Input: part model. Units: mm. Frame: model coordinates. A direction names the side the tool comes from. Coordinates: 2 decimals unless noted, no trailing zeros. Loops run counter-clockwise (first coordinate to the right, second up) from the corner with the lowest first, then second, coordinate; pieces in that order, holes last. Notation, with made-up numbers: (13.25, 4.5) - (68.25, 4.5) arc R23 ccw to (68.25, 26.5) - close; hole circle Ø2 at (-27, -38). An arc over 180 degrees is marked (long way). Use a Markdown table: item, result. Add a question column.
1. Contact query for flat-ended pins moving along their axis: P1, Ø24, axis at x = -31, y = 1.5, coming from the -Z side; P2, Ø2.5, axis at x = -37, y = -3.5, coming from the +Z side; P3, Ø15, axis at y = -4, z = 15.5, coming from the +X side. Output: stop coordinate, or through.
2. Access query for faces 4 (the face through (-39.65, 0.07, 1.01)), 5 (the face through (-22, 0, 2)), 6 (the face through (-30.182, -22.395, 1.014)), 7 (the face through (-35.35, -3.43, 52.99)). Directions: +Z, -Z, +X, -X, +Y, -Y. A direction counts if a zero-diameter tool reaches every point of the face in a straight line with its end or side. Return the directions, or none.
3. Section query B-B on y = -9. Return the cut outline in (x, z), then the cut area to 3 significant figures.
4. Draft query along Z for faces 1 (the face through (-4.69, -8, 1.01)), 2 (the face through (-22, 0, 54)), 3 (the face through (-22, 0, 52)). Return one class per face: released by +Z, released by -Z, zero draft, split by the parting line, or undercut.
5. Section query A-A on x = -2.5. Return the cut outline in (y, z), then the cut area to 3 significant figures.
6. Ray query, L1, parallel to Y at x = -6, z = 1; L2, parallel to Y at x = -37, z = 53; L3, parallel to Z at x = -9, y = 4. Return the intervals inside material, ascending. Write a range as [from, to].
7. Section query D-D on z = 19.5. Return the cut outline in (x, y).
8. Section query C-C on y = 23. Return the cut outline in (x, z).
```python
from build123d import *

# Parameters (mm, degrees)
F1_DEPTH  = 15
F3_D      = 3.3
F5_D      = 3.3
F5_DEPTH  = 13.5
F5_TIP    = 0.9914200214
F7_D      = 3.3
F7_DEPTH  = 13.5
F7_TIP    = 0.9914200214
F9_DEPTH  = 2
F12_D     = 3.3
F12_DEPTH = 13.5
F12_TIP   = 0.9914200214


with BuildPart() as f1:
    # F0 (on Front) → F1 (new body, symmetric)
    with BuildSketch(Plane.XZ):
        Polygon((-45, 0), (0, 0), (0, 2), (-43, 2), (-43, 52), (0, 52), (0, 54), (-45, 54), align=None)
    extrude(amount=F1_DEPTH, both=True)

    # F3 (through all)
    with Locations(Plane(origin=(0, 0, 0), x_dir=(1, 0, 0), z_dir=(0, 0, -1))):
        with Locations((-6, 9), (-6, -9)):
            Hole(F3_D / 2)

    # F5
    with Locations(Plane.XY.offset(54)):
        with Locations((-37, 3.5), (-37, -3.5)):
            Hole(F5_D / 2, depth=F5_DEPTH)
            with Locations((0, 0, -(F5_DEPTH + F5_TIP / 2))):  # 118° drill point
                Cone(0, F5_D / 2, F5_TIP, mode=Mode.SUBTRACT)

    # F7 (one way)
    with BuildSketch(Plane.XY.offset(2)):
        with Locations((-37.9999987781, 0)):
            Circle(F7_D / 2)
    extrude(amount=-F7_DEPTH, mode=Mode.SUBTRACT)
    with Locations(Plane.XY.offset(2)):
        with Locations((-37.9999987781, 0)):
            with Locations((0, 0, -(F7_DEPTH + F7_TIP / 2))):  # 118° drill point
                Cone(0, F7_D / 2, F7_TIP, mode=Mode.SUBTRACT)


with BuildPart() as f9:
    # F8 (on face) → F9 (new body)
    with BuildSketch(Plane.XY.offset(2)):
        Polygon((0, -30), (0, -15), (-43, -15), (-17, -30), align=None)
    extrude(amount=-F9_DEPTH)


with BuildPart() as f9b:
    # F8 (on face) → F9, piece 2 (new body)
    with BuildSketch(Plane.XY.offset(2)):
        Polygon((-17, 30), (-43, 15), (0, 15), (0, 30), align=None)
    extrude(amount=-F9_DEPTH)


with BuildPart() as f1_1:
    add(f1.part)

    # F10: union F9, F9b
    add(f9.part)
    add(f9b.part)

    # F12
    with Locations(Plane.XY.offset(2)):
        with Locations((-9.9999987781, 23), (-9.9999987781, -23)):
            Hole(F12_D / 2, depth=F12_DEPTH)
            with Locations((0, 0, -(F12_DEPTH + F12_TIP / 2))):  # 118° drill point
                Cone(0, F12_D / 2, F12_TIP, mode=Mode.SUBTRACT)


solid = f1_1.part
```
Resolved:
| question | item | result |
|---|---|---|
| 1 | P1 | z = 0 |
| 1 | P2 | z = 2 |
| 1 | P3 | x = -43 |
| 2 | face 4 | -Z |
| 2 | face 5 | +X, +Y, -Y |
| 2 | face 6 | +Z, -Z, -X, -Y |
| 2 | face 7 | +Z |
| 3 | outline | (-45, 0) - (-7.65, 0) - (-7.65, 2) - (-43, 2) - (-43, 52) - (-7.65, 52) - (-7.65, 54) - (-45, 54) - close; (-4.35, 0) - (0, 0) - (0, 2) - (-4.35, 2) - close; (-4.35, 52) - (0, 52) - (0, 54) - (-4.35, 54) - close |
| 3 | area | 267 mm² |
| 4 | face 1 | zero draft |
| 4 | face 2 | released by +Z |
| 4 | face 3 | undercut |
| 5 | outline | (-30, 0) - (30, 0) - (30, 2) - (-30, 2) - close; (-15, 52) - (15, 52) - (15, 54) - (-15, 54) - close |
| 5 | area | 180 mm² |
| 6 | L1 | [-30, -10.65], [-7.35, 7.35], [10.65, 30] |
| 6 | L2 | [-15, -5.15], [-1.85, 1.85], [5.15, 15] |
| 6 | L3 | [0, 2], [52, 54] |
| 7 | outline | (-45, -15) - (-43, -15) - (-43, 15) - (-45, 15) - close |
| 8 | outline | (-29.13, 0) - (-11.65, 0) - (-11.65, 2) - (-29.13, 2) - close; (-8.35, 0) - (0, 0) - (0, 2) - (-8.35, 2) - close |
